Input: dimensioned drawing with shaded views. Units: mm. Origin: part minimum x, y, z. A direction names the side the tool comes from. Round coordinates to 2 decimals unless told otherwise and drop trailing zeros. Loops run counter-clockwise (first coordinate to the right, second up) from the corner with the lowest first, then second, coordinate; pieces in that order, holes last. Notation, with made-up numbers: M 43.5,52 L 53.5,52 A18 ccw 53.5,69 Z; hole C 39,51 d10. An arc over 180 degrees is marked long. Put each result on its own line as item: value. Start each with the question number.
1) Draft query along Y for the marked faces 1, 2, 3 and 4. Return one class per face: +Y half, -Y half, draft (parallel to the pull), parting line (faces both ways), or undercut.
2) Line query: probe 1 along X at (y, z) = (21, 24.45); probe 2 along X at (y, z) = (21, 22.6); probe 3 along Y at (x, z) = (42, 22.7). Output: solid intervals per line, ascending.
3) Section A-A on x = 26. Output: boundary loops of the cut face in (y, z).
4) Section C-C on z = 10.5. Output: boundary loops of the cut face in (x, y).
5) Section D-D on x = 35. Output: boundary loops of the cut face in (y, z), plus the area to 3 significant figures.
6) Pin query (flat end, axial travel): pin 1 (1.8 mm diameter, centred on x = 10, z = 23, fed in from +Y); pin 2 (5 mm diameter, centred on x = 15, y = 9, fed in from -Z); pin 3 (6 mm diameter, centred on x = 27, z = 15, fed in from -Y); pin 4 (10 mm diameter, centred on x = 42, y = 21, fed in from -Z). Return the tip coordinate at first contact, or that it passes through.
7) Section B-B on y = 21. Output: boundary loops of the cut face in (x, z).
8) Reachability of the marked faces 5, 6 and 7 from +Z, -Z, +X, -X, +Y, -Y: full face, straight path, thin tool, end or side. Return the list, or none.
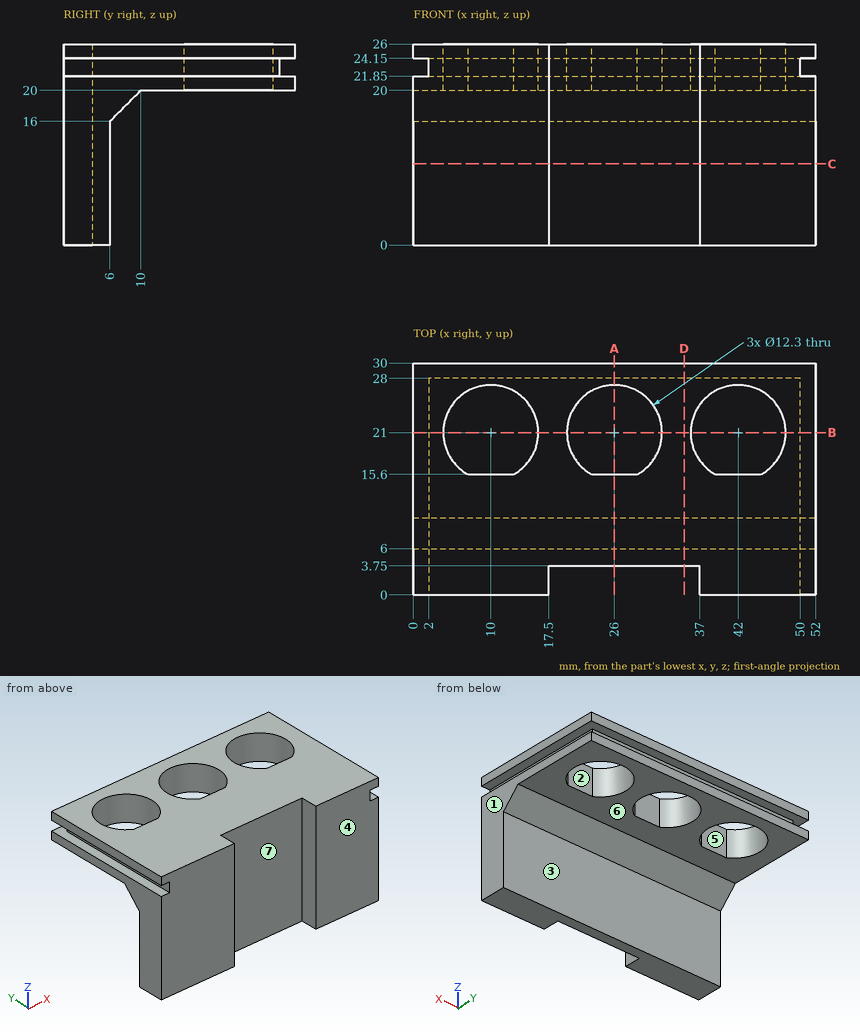
Geometry results:
1. face 1: draft
1. face 2: undercut
1. face 3: +Y half
1. face 4: -Y half
2. probe 1: x = 0 to 3.85, 16.15 to 19.85, 32.15 to 35.85, 48.15 to 52
2. probe 2: x = 2 to 3.85, 16.15 to 19.85, 32.15 to 35.85, 48.15 to 50
2. probe 3: y = 0 to 15.6, 27.15 to 28
3. outline: M 3.75,0 L 6,0 L 6,16 L 10,20 L 15.6,20 L 15.6,26 L 3.75,26 Z; M 27.15,20 L 30,20 L 30,21.85 L 28,21.85 L 28,24.15 L 30,24.15 L 30,26 L 27.15,26 Z
4. outline: M 0,0 L 17.5,0 L 17.5,3.75 L 37,3.75 L 37,0 L 52,0 L 52,6 L 0,6 Z
5. outline: M 3.75,0 L 6,0 L 6,16 L 10,20 L 30,20 L 30,21.85 L 28,21.85 L 28,24.15 L 30,24.15 L 30,26 L 3.75,26 Z
5. area: 206 mm²
6. pin 1: stops at y = 28
6. pin 2: stops at z = 16.5
6. pin 3: stops at y = 3.75
6. pin 4: passes through
7. outline: M 0,20 L 3.85,20 L 3.85,26 L 0,26 L 0,24.15 L 2,24.15 L 2,21.85 L 0,21.85 Z; M 16.15,20 L 19.85,20 L 19.85,26 L 16.15,26 Z; M 32.15,20 L 35.85,20 L 35.85,26 L 32.15,26 Z; M 48.15,20 L 52,20 L 52,21.85 L 50,21.85 L 50,24.15 L 52,24.15 L 52,26 L 48.15,26 Z
8. face 5: +Z, -Z
8. face 6: -Z, +X, -X, +Y
8. face 7: +Z, -Z, -Y
